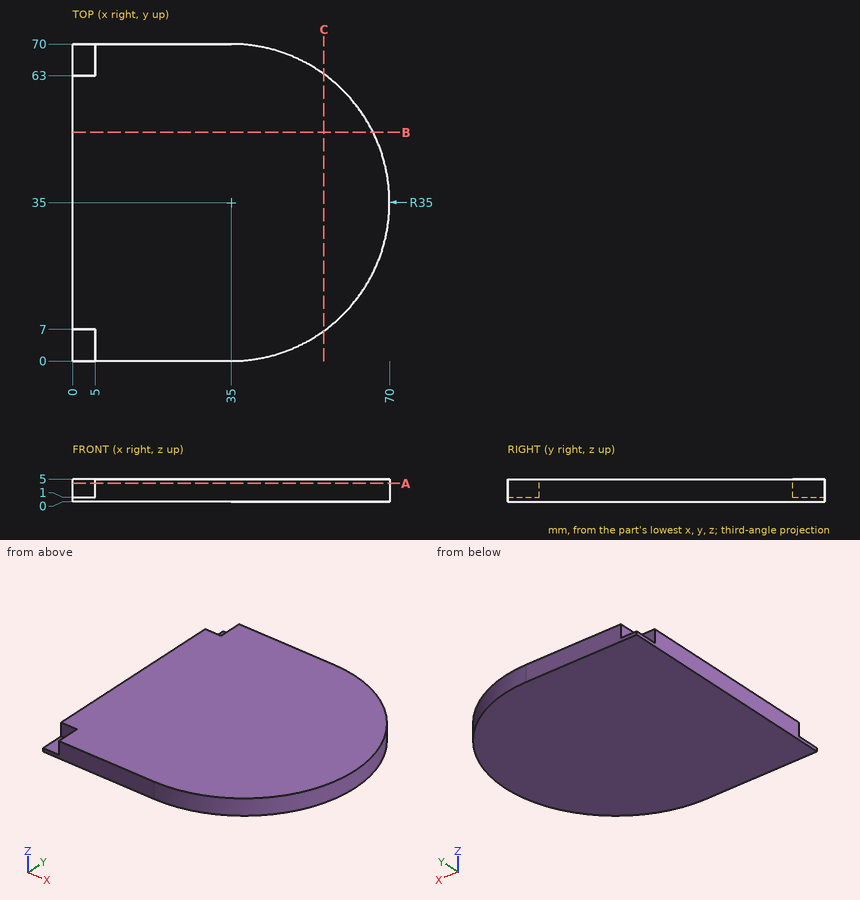
The drawing under review shows one solid part. Ordinate dimensions are in mm from its lowest x, y, z. Give positions to 0.01 mm unless a question says otherwise; leave off trailing zeros. Order: outer loops, then holes, each group sorted by start corner. A loop starts at its lowest first (then second) coordinate and runs counter-clockwise, first axis right, second up. Notation, with made-up numbers: (-17, -28) - (15, -28) arc R24 cw to (15, -17) - close; hole circle Ø2 at (46, 72). An arc over 180 degrees is marked (long way). Answer as a JSON object with one key per item and string values. Group by question number.
Item 1: Take a section at B-B on y = 50.5. Give the boundary of the cut face in (x, z).
Item 2: Take a section at A-A on z = 4.05. Give the boundary of the cut face in (x, y).
Item 3: Take a section at C-C on x = 55.5. Give the boundary of the cut face in (y, z), and give its area (3 significant figures).
Item 4: Clearance check with flat-ended pins moving along their axes: pin 1 Ø4 at (x, y) = (2, 2) entering from +Z; pin 2 Ø2 at (x, z) = (1.5, 2.5) entering from -Y; pin 3 Ø2 at (x, z) = (3.5, 3.5) entering from +Y. State where each tip first meets the part, or that it passes through.
Item 5: Wall thickness on line 1 along Y through (x, z) = (56, 0.8); line 2 along Y through (x, z) = (35.5, 1.15); line 3 along X through (y, z) = (47.5, 3.35): over which ranges is each line inside the solid? List them lowest first.
Reported:
{
 "1": {"outline": "(0, 0) - (66.38, 0) - (66.38, 5) - (0, 5) - close"},
 "2": {"outline": "(0, 7) - (5, 7) - (5, 0) - (35, 0) arc R35 ccw to (35, 70) - (5, 70) - (5, 63) - (0, 63) - close"},
 "3": {"outline": "(6.63, 0) - (63.37, 0) - (63.37, 5) - (6.63, 5) - close", "area": "284 mm^2"},
 "4": {"pin 1": "z = 1", "pin 2": "y = 7", "pin 3": "y = 63"},
 "5": {"line 1": "7 to 63", "line 2": "0 to 70", "line 3": "0 to 67.69"}
}
